from build123d import *

# Parameters (mm, degrees)
F0_W     = 3.5
F0_H     = 170
F3_DEPTH = 15
F5_D     = 3.2
F7_D     = 8


with BuildPart() as f1:
    # F0 (on Front) → F1 (revolve)
    with BuildSketch(Plane.XZ):
        with Locations((10.75, 0)):
            Rectangle(F0_W, F0_H)
        Polygon((9, 90), (9, 85), (12.5, 85), (23, 85), (23, 90), align=None)
        Polygon((12.5, -85), (9, -85), (9, -90), (23, -90), (23, -85), align=None)
    revolve(axis=Axis((0, 0, 0), (0, 0, -1)))

    # F2 (on face) → F3 (join)
    with BuildSketch(Plane(origin=(0, 0, -90), x_dir=(1, 0, 0), z_dir=(0, 0, -1))):
        with BuildLine():
            ThreePointArc((-22.793060873, -3.0783723037), (-22.0098278753, -6.6758877236), (-20.6625952799, -10.1023342006))
            Line((-20.6625952799, -10.1023342006), (20.6625952799, -10.1023342006))
            ThreePointArc((20.6625952799, -10.1023342006), (22.0098278753, -6.6758877236), (22.793060873, -3.0783723037))
            Line((22.793060873, -3.0783723037), (4, -3.0783723037))
            Line((4, -3.0783723037), (4, -5.0783723037))
            Line((4, -5.0783723037), (-4, -5.0783723037))
            Line((-4, -5.0783723037), (-4, -3.0783723037))
            Line((-4, -3.0783723037), (-22.793060873, -3.0783723037))
        make_face()
    extrude(amount=F3_DEPTH)

    # F5 (through all)
    with Locations(Plane.XZ.offset(-3.0783723037)):
        with Locations((-7.4993308043, -95), (7.5006691957, -95)):
            Hole(F5_D / 2)

    # F7 (through all)
    with Locations(Plane.XY.offset(90)):
        with Locations((-14.2894191624, -8.25), (0, 16.5), (14.2894191624, -8.25)):
            Hole(F7_D / 2)


solid = f1.part
CAD build for the part. Positions are in the model's coordinates, mm. A direction names the side the tool comes from. Coordinates: 2 decimals unless noted, no trailing zeros. Order: outer loops, then holes, each group sorted by start corner. A loop starts at its lowest first (then second) coordinate and runs counter-clockwise, first axis right, second up.
Item 1: Band-saw the part on A-A on z = -19. List the corners of the cut face in (x, y), plus the area to 3 significant figures.
Check sheet entries:
outline: circle Ø25 at (0, 0); hole circle Ø18 at (0, 0)
area: 236 mm2
Item 2: 3-axis set-ups, long thin cutter, end or side, ignore diameter. For faces 4 (the face through (-13, 3.078, -97)), 5 (the face through (0, 5.078, -97)), 6 (the face through (-10, 10, 85)): which of +Z, -Z, +X, -X, +Y, -Y reach the whole face in a straight line?
Check sheet entries:
face 4: -Z, +X, -X, -Y
face 5: +Z, -Z, -Y
face 6: none
Item 3: Drill centre lines: L1, parallel to Y at x = 0, z = -21; L2, parallel to Z at x = -12.5, y = -15.5; L3, parallel to Z at x = -14.5, y = 9. Where is each one in solid material? Low to high.
Check sheet entries:
L1: y = -12.5 to -9, 9 to 12.5
L2: z = -90 to -85, 85 to 90
L3: z = -105 to -85, 85 to 90
Item 4: Two-plate mould, pull along Z, no slides. Class faces 1 (the face through (11.923, -3.755, 1.19)), 2 (the face through (0, 12, -90)), 3 (the face through (14, 3.078, -97)): +Z half, -Z half, draft (parallel to the pull), parting line (faces both ways), or undercut.
Check sheet entries:
face 1: undercut
face 2: -Z half
face 3: draft
Item 5: Pin check, flat tips, straight feed: pin 1 Ø4 at (x, y) = (-9, 14) entering from -Z; pin 2 Ø6 at (y, z) = (0.5, 33) entering from -X; pin 3 Ø2 at (y, z) = (-7, -70) entering from -X. Stop position of each tip, or through.
Check sheet entries:
pin 1: stops at z = -90
pin 2: stops at x = -12.5
pin 3: stops at x = -10.97
